CAD build for the part. Positions are in the model's coordinates, mm. Face numbers are marked on the shaded views. Give positions to 0.01 mm unless a question says otherwise; leave off trailing zeros. Loops run counter-clockwise (first coordinate to the right, second up) from the corner with the lowest first, then second, coordinate; pieces in that order, holes last.
```python
from build123d import *

# Parameters (mm, degrees)
SKETCH2_R           = 0.5
SKETCH2_R_2         = 0.507316736
SKETCH2_R_3         = 0.412242995
BOSS_EXTRUDE1_DEPTH = 3
FILLET1_R           = 3


with BuildPart() as part:
    # Sketch2 → Boss-Extrude1 (new body)
    with BuildSketch(Plane.XY):
        Polygon((-11, 4.5), (11, 4.5), (11, 0.5), (11, -0.5), (11, -4.5), (-11, -4.5), (-11, -1.5), (-8, -1.5), (-8, 1.5), (-11, 1.5), align=None)
        with Locations((7, 0)):
            Circle(SKETCH2_R, mode=Mode.SUBTRACT)
        with Locations((3, 0)):
            Circle(SKETCH2_R_2, mode=Mode.SUBTRACT)
        with Locations((-5, 0)):
            Circle(SKETCH2_R_3, mode=Mode.SUBTRACT)
    extrude(amount=BOSS_EXTRUDE1_DEPTH)

    # Fillet1
    fillet1_edges = [part.edges().sort_by_distance(p)[0] for p in [
        (11, -4.5, 1.5),
        (11, 4.5, 1.5),
    ]]
    fillet(fillet1_edges, radius=FILLET1_R)


solid = part.part
```
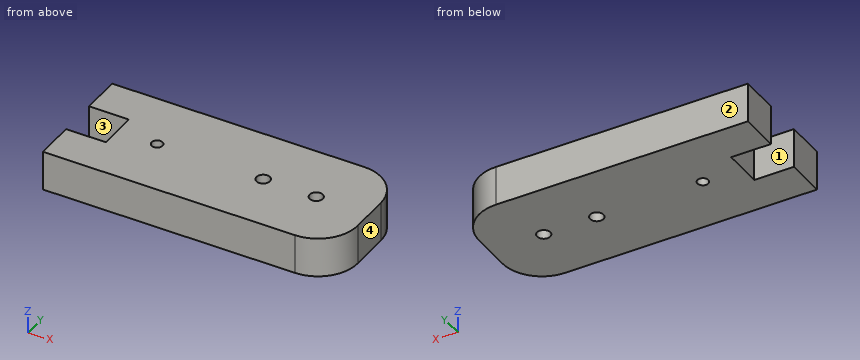
1. Drop flat-ended pins along their axis: pin 1 (1.5 mm diameter, centred on x = -5.5, y = 1.5, fed in from -Z); pin 2 (1.5 mm diameter, centred on y = 0.5, z = 2, fed in from -X). Give the stop position or say it passes through.
Responses:
pin 1: stops at z = 0
pin 2: stops at x = -8
2. Saw through at C-C, the plane z = 2.45. List the corners of the cut face in (x, y).
Responses:
outline: (-11, -4.5) - (8, -4.5) arc R3 ccw to (11, -1.5) - (11, 1.5) arc R3 ccw to (8, 4.5) - (-11, 4.5) - (-11, 1.5) - (-8, 1.5) - (-8, -1.5) - (-11, -1.5) - close; hole circle Ø0.82 at (-5, 0); hole circle Ø1.01 at (3, 0); hole circle Ø1 at (7, 0)
3. Pull direction Y, two halves, no side cores. Call the marked faces 1, 2, 3 and 4: released by +Y, released by -Y, zero draft, split by the parting line, or undercut.
Responses:
face 1: undercut
face 2: released by +Y
face 3: undercut
face 4: zero draft
4. Probe line 1 along X through (y, z) = (0.25, 2.15); line 2 along Y through (x, z) = (-8.5, 2.4); line 3 along Y through (x, z) = (7, 1.55). List the from-to ranges inside material, lowest first.
Responses:
line 1: x = -8 to -5.33, -4.67 to 2.56, 3.44 to 6.57, 7.43 to 11
line 2: y = -4.5 to -1.5, 1.5 to 4.5
line 3: y = -4.5 to -0.5, 0.5 to 4.5
5. Saw through at D-D, the plane x = 7. List the corners of the cut face in (y, z).
Responses:
outline: (-4.5, 0) - (-0.5, 0) - (-0.5, 3) - (-4.5, 3) - close; (0.5, 0) - (4.5, 0) - (4.5, 3) - (0.5, 3) - close
6. Saw through at B-B, the plane y = 0. List the corners of the cut face in (x, z).
Responses:
outline: (-8, 0) - (-5.41, 0) - (-5.41, 3) - (-8, 3) - close; (-4.59, 0) - (2.49, 0) - (2.49, 3) - (-4.59, 3) - close; (3.51, 0) - (6.5, 0) - (6.5, 3) - (3.51, 3) - close; (7.5, 0) - (11, 0) - (11, 3) - (7.5, 3) - close
7. Saw through at A-A, the plane x = -5. List the corners of the cut face in (y, z).
Responses:
outline: (-4.5, 0) - (-0.41, 0) - (-0.41, 3) - (-4.5, 3) - close; (0.41, 0) - (4.5, 0) - (4.5, 3) - (0.41, 3) - close
